Source: CAD feature listing. Evaluate the final solid. Frame: model axes, mm. A direction names the side the tool comes from. Coordinates: 2 decimals unless noted, no trailing zeros. Write each loop counter-clockwise with the first axis right and the second up, starting at its lowest first coordinate (ties: lowest second). Pieces come first, ordered by that corner, then holes. Notation, with made-up numbers: M 55.5,69.5 L 66.5,69.5 A21 ccw 66.5,77.5 Z; hole C 25.25,50 d7. An arc over 180 degrees is marked long. One line per item, written item: value. Start each with the question number.
Item 1: Cut plane C-C, the plane y = 110. Output: boundary loops of the cut face in (x, z).
Item 2: Cut plane B-B, the plane z = 215.9. Output: boundary loops of the cut face in (x, y), then the cut area to 3 significant figures.
Item 3: Pin query (flat end, axial travel): P1, Ø4, axis at x = 1273, z = 322, coming from the -Y side. Return the tip coordinate at first contact, or that it passes through.
Item 4: Cut plane D-D, the plane x = 90. Output: boundary loops of the cut face in (y, z), then the cut area to 3 significant figures.
Item 5: Cut plane A-A, the plane y = -120.5. Output: boundary loops of the cut face in (x, z), then the cut area to 3 significant figures.
Item 6: Mould query, pull axis X, two halves, no side actions, for faces 1 (the flat face through (2032, 111, 214)), 2 (the flat face through (2032, 38, 404)), 3 (the flat face through (-62.078, 2, 214)). Classes: released by +X, released by -X, zero draft, split by the parting line, or undercut.
Item 7: Ray query, L1, parallel to X at y = -64.5, z = 340; L2, parallel to Y at x = 443, z = 152.5; L3, parallel to X at y = 73.5, z = 40. Return the intervals inside material, ascending. Write a range as from..to.
Item 8: Set-up query: faces 4 (the cylindrical face through (2062.609, -159.755, 180.431)), 5 (the flat face through (2032, -62, 214)), 6 (the flat face through (1030, 76.2, 219)). Return all of +Z, -Z, +X, -X, +Y, -Y with unobstructed straight access to the full face (end or side cutting, diameter ignored); none if empty.
Autodesk Inventor part; units mm, degrees
ref_plane "YZ Plane" through (0, 0, 0) normal (1, 0, 0) x (0, 1, 0)
ref_plane "XZ Plane" through (0, 0, 0) normal (0, 1, 0) x (-1, 0, 0)
ref_plane "XY Plane" through (0, 0, 0) normal (0, 0, 1) x (1, 0, 0)
sketch "Sketch1" plane through (0, 0, 0) normal (0, 1, 0) x (-1, 0, 0)
  line L0 (0, 0) -> (-2032, 0)
  line L1 (-2032, 0) -> (-2032, 431.8)
  line L2 (-2032, 431.8) -> (0, 431.8)
  line L3 (0, 431.8) -> (0, 0)
  dimension "d0" = 2032
  dimension "d1" = 431.8
extrude "Extrusion1" add sketch "Sketch1" along normal blind 76.2
sketch "Sketch2" plane through (0, 0, 0) normal (0, -1, 0) x (1, 0, 0)
  line L0 (2094.0877, 379.5522) -> (2032, 379.5522)
  line L1 (2032, 0) -> (0, 0)
  line L2 (0, 431.8) -> (2032, 431.8)
  line L3 (-62.0877, 379.5522) -> (0, 379.5522)
  line L4 (2094.0877, 215.9061) -> (2032, 215.9061)
  line L5 (0, 215.9) -> (-62.0877, 215.9061)
  line L6 (2094.0877, 379.5522) -> (2094.0877, 215.9061)
  line L7 (2032, 215.9061) -> (2032, 379.5522)
  line L8 (2032, 431.8) -> (2032, 0)
  line L9 (0, 215.9) -> (0, 379.5522)
  line L10 (0, 0) -> (0, 431.8)
  line L11 (-62.0877, 215.9061) -> (-62.0877, 379.5522)
  point P0 (2063.0438, 379.5522)
revolve "Revolution1" add sketch "Sketch2" angle 360 about axis through (2094.0877, 0, 215.9061) along (-1, 0, 0) contours L6 L4 L7 L0
sketch "Sketch3" plane through (0, 0, 0) normal (0, -1, 0) x (1, 0, 0)
  line L0 (0, 215.9) -> (-62.0776, 215.9)
  line L1 (0, 431.8) -> (2032, 431.8)
  line L2 (0, 431.8) -> (0, 379.5522)
  line L3 (0, 215.9) -> (0, 379.5522)
  line L4 (-62.0776, 215.9) -> (-62.0776, 379.5522)
  line L5 (-62.0776, 379.5522) -> (0, 379.5522)
  point P0 (-31.0388, 431.8)
  dimension "d7" = 62.0776
  dimension "d10" = 215.9
revolve "Revolution2" add sketch "Sketch3" angle 360 about axis through (0, 0, 215.9) along (-1, 0, 0)
properties part number "Solor Cleaner - Solor Panal Bace"
From the geometry:
1. outline: M -62.08,94.73 L 0,94.73 L 0,337.07 L -62.08,337.07 Z; M 2032,94.74 L 2094.09,94.74 L 2094.09,337.07 L 2032,337.07 Z
2. outline: M -62.08,-163.65 L 0,-163.65 L 0,0 L 2032,0 L 2032,-163.65 L 2094.09,-163.65 L 2094.09,163.65 L 2032,163.65 L 2032,76.2 L 0,76.2 L 0,163.65 L -62.08,163.65 Z
2. area: 195,000 mm²
3. P1: stops at y = 0
4. outline: M 0,0 L 76.2,0 L 76.2,431.8 L 0,431.8 Z
4. area: 32,900 mm²
5. outline: M -62.08,105.17 L 0,105.17 L 0,326.63 L -62.08,326.63 Z; M 2032,105.18 L 2094.09,105.18 L 2094.09,326.63 L 2032,326.63 Z
5. area: 27,500 mm²
6. face 1: undercut
6. face 2: released by +X
6. face 3: released by -X
7. L1: x = -62.08..0, 2032..2094.09
7. L2: y = 0..76.2
7. L3: x = 0..2032
8. face 4: +X
8. face 5: +Z, -Z, -Y
8. face 6: +Z, -Z, +Y
